The listing builds one solid part. Answer for the finished solid, in the listing's coordinates (mm). Face numbers are marked on the shaded views. A direction names the side the tool comes from. Round coordinates to 2 decimals unless told otherwise and drop trailing zeros. Write each loop counter-clockwise with the first axis right and the second up, starting at its lowest first coordinate (ties: lowest second). Pieces come first, ordered by that corner, then holes.
(1) A cutting plane is placed at A-A, the plane y = 50.8. Give the vertices of the cut face in (x, z) (3 decimals).
(2) A cutting plane is placed at D-D, the plane z = 20.5. Give the vertices of the cut face in (x, y) (3 decimals), and give its area (3 significant figures).
(3) A cutting plane is placed at B-B, the plane x = 12.7. Give the vertices of the cut face in (y, z) (3 decimals), and give its area (3 significant figures).
(4) A cutting plane is placed at C-C, the plane z = 12.7. Give the vertices of the cut face in (x, y) (3 decimals).
(5) Find the intervals of material crossed by probe 1 along Z at (x, y) = (12.7, 1.2); probe 2 along Y at (x, z) = (0.7, 12.7) (3 decimals), in increasing order.
(6) For the marked faces 1 and 2, determine the directions among +Z, -Z, +X, -X, +Y, -Y from which every point of the face is accessible in a straight line to the end or side of a thin tool.
(7) Each of these flat-tipped pins is pushed along its axis until it touches: pin 1 Ø10 at (y, z) = (26.5, 9.5) entering from -X; pin 2 Ø7.5 at (y, z) = (50.8, 12.7) entering from +X (3 decimals); pin 3 Ø11 at (x, z) = (11, 9) entering from +Y (3 decimals). Where does it stop, or does it pass through?
from build123d import *

# Parameters (mm, degrees)
BOSS_EXTRUDE1_DEPTH            = 25.4
SKETCH2_R                      = 3.175
CUT_EXTRUDE1_DEPTH             = 26.4
F_9_0_196_DIAMETER_HOLE1_D     = 4.9784
F_9_0_196_DIAMETER_HOLE1_DEPTH = 3.175


with BuildPart() as part:
    # Sketch1 → Boss-Extrude1 (new body)
    with BuildSketch(Plane.XY):
        Polygon((0, 0), (0, 63.5), (3.175, 63.5), (3.175, 3.175), (25.4, 3.175), (25.4, 0), align=None)
    extrude(amount=BOSS_EXTRUDE1_DEPTH)

    # Sketch2 → Cut-Extrude1 (cut, through all)
    with BuildSketch(Plane.ZY):
        with Locations((12.7, 50.8)):
            Circle(SKETCH2_R)
    extrude(amount=-CUT_EXTRUDE1_DEPTH, mode=Mode.SUBTRACT)

    # #9 (0.196) Diameter Hole1
    with Locations(Plane(origin=(0, 0, 0), x_dir=(-1, 0, 0), z_dir=(0, -1, 0))):
        with Locations((-12.7, -12.7)):
            Hole(F_9_0_196_DIAMETER_HOLE1_D / 2, depth=F_9_0_196_DIAMETER_HOLE1_DEPTH)


solid = part.part
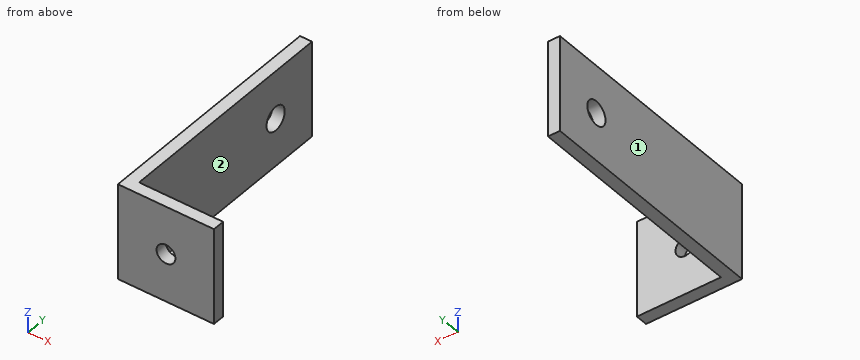
Solutions:
1. outline: (0, 0) - (3.175, 0) - (3.175, 9.525) - (0, 9.525) - close; (0, 15.875) - (3.175, 15.875) - (3.175, 25.4) - (0, 25.4) - close
2. outline: (0, 0) - (25.4, 0) - (25.4, 3.175) - (3.175, 3.175) - (3.175, 63.5) - (0, 63.5) - close
2. area: 272 mm2
3. outline: (0, 0) - (3.175, 0) - (3.175, 10.211) - (0, 10.211) - close; (0, 15.189) - (3.175, 15.189) - (3.175, 25.4) - (0, 25.4) - close
3. area: 64.8 mm2
4. outline: (0, 0) - (10.211, 0) - (10.211, 3.175) - (3.175, 3.175) - (3.175, 47.625) - (0, 47.625) - close; (0, 53.975) - (3.175, 53.975) - (3.175, 63.5) - (0, 63.5) - close; (15.189, 0) - (25.4, 0) - (25.4, 3.175) - (15.189, 3.175) - close
5. probe 1: z = 0 to 10.21, 15.19 to 25.4
5. probe 2: y = 0 to 47.625, 53.975 to 63.5
6. face 1: +Z, -Z, -X, +Y, -Y
6. face 2: +Z, -Z, +X, +Y
7. pin 1: stops at x = 0
7. pin 2: stops at x = 3.175
7. pin 3: stops at y = 3.175
